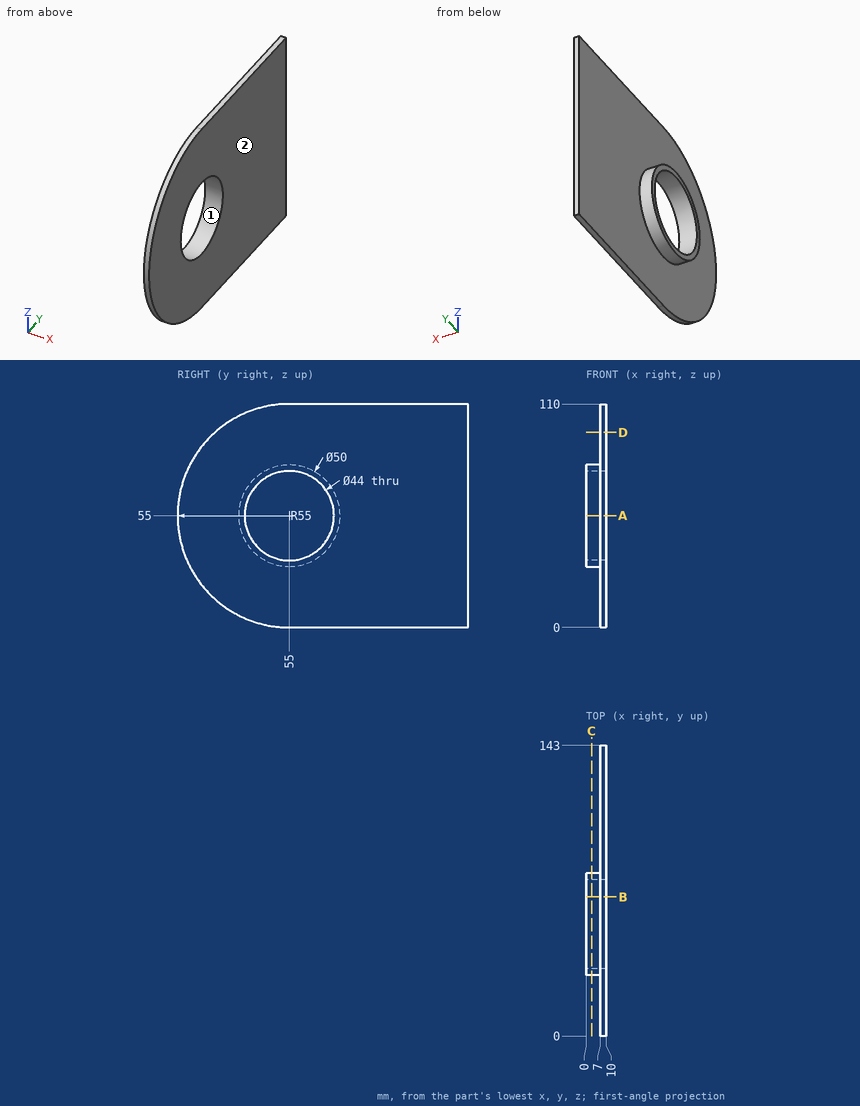
Study the drawing (mm; zero at the part's minimum x, y, z) and answer. Give positions to 0.01 mm unless a question says otherwise; leave off trailing zeros. Loops run counter-clockwise (first coordinate to the right, second up) from the corner with the lowest first, then second, coordinate; pieces in that order, holes last. Notation, with made-up numbers: (33.5, 70) -> (51.5, 70) arc R25 ccw to (51.5, 94) -> close; hole circle Ø9 at (66.5, 69). An arc over 180 degrees is marked (long way). Write item = value, one per line. Start each with the question number.
(1) Find section A-A on z = 55. Give the vertices of the cut face in (x, y), and give its area (3 significant figures).
(2) Find section C-C on x = 2.75. Give the vertices of the cut face in (y, z).
(3) The mould has two halves that part along Y. Classify the marked faces 1 and 2: +Y half, -Y half, draft (parallel to the pull), parting line (faces both ways), or undercut.
(4) Given pin 1 Ø4 at (x, z) = (2, 31) entering from +Y; pin 2 Ø4 at (x, z) = (8.5, 26) entering from -Y; pin 3 Ø3 at (y, z) = (103.5, 48.5) entering from -X, each flat-ended and moving along its own axis, determine where each tip first touches the part or whether it passes through.
(5) Find section B-B on y = 68.5. Give the vertices of the cut face in (x, z).
(6) Find section D-D on z = 96. Give the vertices of the cut face in (x, y), and give its area (3 significant figures).
(7) Find the intervals of material crossed by probe 1 along Y at (x, z) = (7.75, 55); probe 2 along Y at (x, z) = (4.5, 55); probe 3 along X at (y, z) = (21.5, 71.5), in increasing order. Write a range as from..to.
From the geometry:
q1.outline = (0, 30) -> (7, 30) -> (7, 0) -> (10, 0) -> (10, 33) -> (0, 33) -> close; (0, 77) -> (10, 77) -> (10, 143) -> (7, 143) -> (7, 80) -> (0, 80) -> close
q1.area = 339 mm^2
q2.outline = circle Ø50 at (55, 55); hole circle Ø44 at (55, 55)
q3.face_1 = undercut
q3.face_2 = draft
q4.pin_1 = 66.87
q4.pin_2 = 7.08
q4.pin_3 = 7
q5.outline = (0, 33.96) -> (7, 33.96) -> (7, 0) -> (10, 0) -> (10, 37.63) -> (0, 37.63) -> close; (0, 72.37) -> (10, 72.37) -> (10, 110) -> (7, 110) -> (7, 76.04) -> (0, 76.04) -> close
q6.outline = (7, 18.34) -> (10, 18.34) -> (10, 143) -> (7, 143) -> close
q6.area = 374 mm^2
q7.probe_1 = 0..33, 77..143
q7.probe_2 = 30..33, 77..80
q7.probe_3 = 7..10
